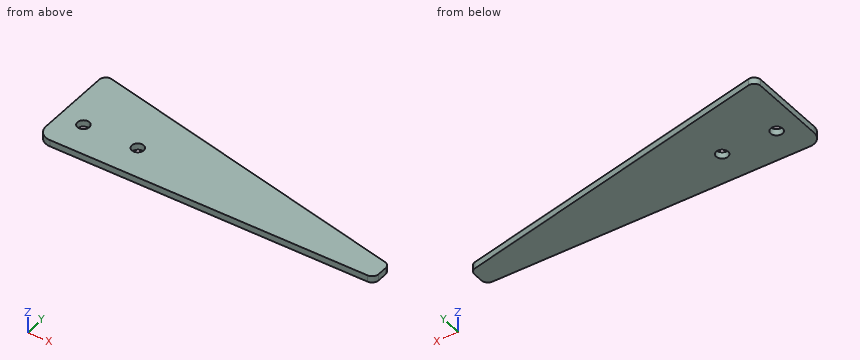
```python
from build123d import *

# Parameters (mm, degrees)
BASE_FLANGE1_DEPTH = 3
SKETCH6_R          = 2.75
CUT_EXTRUDE1_DEPTH = 10


# Sheet-metal steps are written as plain solids
with BuildPart() as part:
    # Sketch1 → Base-Flange1 (new body)
    with BuildSketch(Plane.XY):
        with BuildLine():
            Line((6, 0), (152, 0))
            ThreePointArc((152, 0), (154.121320344, 0.878679656), (155, 3))
            Line((155, 3), (155, 7.601887371))
            ThreePointArc((155, 7.601887371), (154.343325398, 9.475073448), (152.660782614, 10.528210377))
            Line((152.660782614, 10.528210377), (3.660782614, 44.173371668))
            ThreePointArc((3.660782614, 44.173371668), (1.126813923, 43.59037406), (0, 41.247048662))
            Line((0, 41.247048662), (0, 6))
            ThreePointArc((0, 6), (1.757359313, 1.757359313), (6, 0))
        make_face()
    extrude(amount=-BASE_FLANGE1_DEPTH)

    # Sketch6 → Cut-Extrude1 (cut)
    with BuildSketch(Plane(origin=(0, 0, -3), x_dir=(-1, 0, 0), z_dir=(0, 0, -1))):
        with Locations((-11, 15)):
            Circle(SKETCH6_R)
        with Locations((-36, 15)):
            Circle(SKETCH6_R)
    extrude(amount=-CUT_EXTRUDE1_DEPTH, mode=Mode.SUBTRACT)


solid = part.part
```
For this review, take the finished solid that the model builds, in its own axes (mm). Round coordinates to 2 decimals unless told otherwise and drop trailing zeros. Write each loop counter-clockwise with the first axis right and the second up, starting at its lowest first coordinate (ties: lowest second). Pieces come first, ordered by that corner, then holes. Notation, with made-up numbers: (45, 48) - (57, 48) arc R24 cw to (57, 78) - close; hole circle Ø10 at (-13.75, 76). An arc over 180 degrees is marked (long way). Answer as a JSON object with one key per item and string values.
1. We need section C-C on y = 15. Give the boundary of the cut face in (x, z).
Response values:
{"outline": "(0, -3) - (8.25, -3) - (8.25, 0) - (0, 0) - close; (13.75, -3) - (33.25, -3) - (33.25, 0) - (13.75, 0) - close; (38.75, -3) - (132.86, -3) - (132.86, 0) - (38.75, 0) - close"}
2. To check wall thickness, follow line 1 along Y through (x, z) = (11, -2.4); line 2 along Y through (x, z) = (52, -0.8); line 3 along Y through (x, z) = (36, -0.95). State the ranges of each line that lie inside material, in increasing order.
Response values:
{"line 1": "y = 0 to 12.25, 17.75 to 42.52", "line 2": "y = 0 to 33.26", "line 3": "y = 0 to 12.25, 17.75 to 36.87"}
3. We need section D-D on x = 36. Give the boundary of the cut face in (y, z), then the cut area to 3 significant figures.
Response values:
{"outline": "(0, -3) - (12.25, -3) - (12.25, 0) - (0, 0) - close; (17.75, -3) - (36.87, -3) - (36.87, 0) - (17.75, 0) - close", "area": "94.1 mm2"}
4. We need section A-A on z = -2. Give the boundary of the cut face in (x, y).
Response values:
{"outline": "(0, 6) arc R6 ccw to (6, 0) - (152, 0) arc R3 ccw to (155, 3) - (155, 7.6) arc R3 ccw to (152.66, 10.53) - (3.66, 44.17) arc R3 ccw to (0, 41.25) - close; hole circle Ø5.5 at (11, 15); hole circle Ø5.5 at (36, 15)"}
5. We need section B-B on x = 11. Give the boundary of the cut face in (y, z).
Response values:
{"outline": "(0, -3) - (12.25, -3) - (12.25, 0) - (0, 0) - close; (17.75, -3) - (42.52, -3) - (42.52, 0) - (17.75, 0) - close"}
6. For pin 1 Ø5 at (x, y) = (11, 15) entering from +Z, flat-tipped, find the tip position at first contact; note if it passes through.
Response values:
{"pin 1": "passes through"}
